from build123d import *

# Parameters (mm, degrees)
ESQUISSE2_R        = 2
BOSS_EXTRU_1_DEPTH = 6
BOSS_EXTRU_2_DEPTH = 25


with BuildPart() as part:
    # Esquisse1 → Révolution4 (revolve)
    with BuildSketch(Plane.XY):
        Polygon((-5.618645861, -7.271198097), (35.881354139, -7.271198097), (35.881354139, -1.271198097), (-0.618645861, -1.271198097), (-0.618645861, 18.728801903), (-14.118645861, 18.728801903), (-14.118645861, 14.081661898), (-5.618645861, 14.081661898), align=None)
    revolve(axis=Axis((-14.118645861, 18.728801903, 0), (0, -1, 0)))

    # Esquisse2 → Boss.-Extru.1 (add)
    with BuildSketch(Plane(origin=(0, -1.271198097, 0), x_dir=(1, 0, 0), z_dir=(0, 1, 0))):
        with Locations((-14.118645861, -25)):
            Circle(ESQUISSE2_R)
        with Locations((-14.118645861, 25)):
            Circle(ESQUISSE2_R)
    extrude(amount=BOSS_EXTRU_1_DEPTH)

    # Esquisse3 → Boss.-Extru.2 (add)
    with BuildSketch(Plane.XZ.offset(7.271198097)):
        with BuildLine():
            ThreePointArc((-7.618645861, -5.477225575), (-6.13428615, -2.915475947), (-5.618645861, 0))
            ThreePointArc((-5.618645861, 0), (-6.13428615, 2.915475947), (-7.618645861, 5.477225575))
            Line((-7.618645861, 5.477225575), (-7.618645861, 0))
            Line((-7.618645861, 0), (-7.618645861, -5.477225575))
        make_face()
    extrude(amount=-BOSS_EXTRU_2_DEPTH)


solid = part.part
Input: part model. Units: mm. Frame: model coordinates. A direction names the side the tool comes from. Give positions to 0.01 mm unless a question says otherwise; leave off trailing zeros. Write each loop counter-clockwise with the first axis right and the second up, starting at its lowest first coordinate (ties: lowest second). Pieces come first, ordered by that corner, then holes. Notation, with made-up numbers: (-15.75, 32) -> (2.25, 32) arc R22 cw to (2.25, 70) -> close; hole circle Ø1 at (23, -23). An arc over 180 degrees is marked (long way). Use one line per item in the form item = value. Start each with the question number.
1) Ray query, probe 1 along Z at (x, y) = (-14.5, 3.75); probe 2 along Y at (x, z) = (-6, -25); probe 3 along Y at (x, z) = (-18, 6). Return the intervals inside material, ascending. Write a range as from..to.
2) Section query D-D on z = -25. Return the cut outline in (x, y), then the cut area to 3 significant figures.
3) Section query A-A on y = 3.5. Return the cut outline in (x, z).
4) Section query B-B on z = 0. Return the cut outline in (x, y), then the cut area to 3 significant figures.
5) Section query C-C on x = -13.5. Return the cut outline in (y, z), then the cut area to 3 significant figures.
6) Set-up query: faces 1 (the flat face through (-14, 18.729, 0)), 2 (the cylindrical face through (-14.552, 1.687, -23.048)), 3 (the flat face through (-15, -7.271, -10)), 4 (the flat face through (-7.619, 3, 0)), 5 (the flat face through (-14, 4.729, -25)). Return all of +Z, -Z, +X, -X, +Y, -Y with unobstructed straight access to the full face (end or side cutting, diameter ignored); none if empty.
7) Pin query (flat end, axial travel): pin 1 (1.2 mm diameter, centred on x = -14.5, z = 24, fed in from +Y); pin 2 (4 mm diameter, centred on x = 17.5, z = -25, fed in from +Y); pin 3 (10 mm diameter, centred on x = -1.5, y = 4, fed in from -Z). Return the tip coordinate at first contact, or that it passes through.
8) Draft query along X for faces 6 (the cylindrical face through (-22.614, 3.256, 0.29)), 7 (the flat face through (-14, 4.729, 25)), 8 (the cylindrical face through (-15.706, 1.687, 26.217)). Return one class per face: pulls with the +X half, pulls with the -X half, needs draft (parallel to the pull), parting line crosses it, or undercut.
Outcome:
q1.probe_1 = -26.96..-23.04, -13.49..-8.49, 8.49..13.49, 23.04..26.96
q1.probe_2 = -7.27..-1.27
q1.probe_3 = 14.08..18.73
q2.outline = (-57.42, -7.27) -> (29.18, -7.27) -> (29.18, -1.27) -> (-12.12, -1.27) -> (-12.12, 4.73) -> (-16.12, 4.73) -> (-16.12, -1.27) -> (-57.42, -1.27) -> close
q2.area = 544 mm^2
q3.outline = circle Ø27 at (-14.12, 0); circle Ø4 at (-14.12, -25); circle Ø4 at (-14.12, 25); hole (-7.62, -5.48) -> (-7.62, 5.48) arc R8.5 ccw (long way) to start
q4.outline = (-64.12, -7.27) -> (-22.62, -7.27) -> (-22.62, 14.08) -> (-7.62, 14.08) -> (-7.62, -7.27) -> (35.88, -7.27) -> (35.88, -1.27) -> (-0.62, -1.27) -> (-0.62, 18.73) -> (-27.62, 18.73) -> (-27.62, -1.27) -> (-64.12, -1.27) -> close
q4.area = 820 mm^2
q5.outline = (-7.27, -50) -> (-1.27, -50) -> (-1.27, -26.9) -> (4.73, -26.9) -> (4.73, -23.1) -> (-1.27, -23.1) -> (-1.27, -13.49) -> (18.73, -13.49) -> (18.73, 13.49) -> (-1.27, 13.49) -> (-1.27, 23.1) -> (4.73, 23.1) -> (4.73, 26.9) -> (-1.27, 26.9) -> (-1.27, 50) -> (-7.27, 50) -> (-7.27, 8.48) -> (14.08, 8.48) -> (14.08, -8.48) -> (-7.27, -8.48) -> close
q5.area = 823 mm^2
q6.face_1 = +Z, -Z, +X, -X, +Y
q6.face_2 = +Y
q6.face_3 = +Z, -Z, +X, -X, -Y
q6.face_4 = -Y
q6.face_5 = -Z, +X, -X, +Y
q7.pin_1 = 4.73
q7.pin_2 = -1.27
q7.pin_3 = -11.14
q8.face_6 = undercut
q8.face_7 = needs draft
q8.face_8 = parting line crosses it
